The listing builds one solid part. Answer for the finished solid, in the listing's coordinates (mm). A direction names the side the tool comes from. Round coordinates to 2 decimals unless told otherwise and drop trailing zeros. Write each loop counter-clockwise with the first axis right and the second up, starting at its lowest first coordinate (ties: lowest second). Pieces come first, ordered by that corner, then holes.
(1) The mould has two halves that part along Y. Classify faces 5 (the face through (7.013, -0.356, 44.539)), 6 (the face through (72.38, 21.78, 6.44)), 7 (the face through (72.38, -21.78, 6.44)), 8 (the face through (29.1, -2.93, 7.066)): +Y half, -Y half, draft (parallel to the pull), parting line (faces both ways), or undercut.
(2) A cutting plane is placed at A-A, the plane x = 27. Give the vertices of the cut face in (y, z).
(3) A cutting plane is placed at D-D, the plane y = -9. Give the vertices of the cut face in (x, z).
(4) Find the intervals of material crossed by probe 1 along Z at (x, y) = (28, 0); probe 2 along Z at (x, y) = (43, 0); probe 3 along X at (y, z) = (8.5, 15), in increasing order.
(5) A cutting plane is placed at C-C, the plane z = 36. Give the vertices of the cut face in (x, y), and give its area (3 significant figures).
(6) A cutting plane is placed at B-B, the plane y = 0. Give the vertices of the cut face in (x, z), and give its area (3 significant figures).
(7) For faces 1 (the face through (25.4, -19, 38)), 2 (the face through (25.4, 19, 38)), 3 (the face through (24, -25.4, 20)), 4 (the face through (64, 16, 12.7)), determine the directions among +Z, -Z, +X, -X, +Y, -Y from which every point of the face is accessible in a straight line to the end or side of a thin tool.
(8) Each of these flat-tipped pins is pushed along its axis until it touches: pin 1 Ø20.5 at (x, z) = (34.5, 32.5) entering from +Y; pin 2 Ø12.5 at (x, z) = (40.5, 35.5) entering from -Y; pin 3 Ø4 at (x, y) = (32, -20) entering from +Z; pin 4 Ø6.5 at (x, y) = (45.5, -4) entering from +Z. Where does it stop, or does it pass through?
from build123d import *

# Parameters (mm, degrees)
F1_DEPTH = 25.4
F2_DEPTH = 12.7
F3_R     = 6.35
F4_DEPTH = 76.201
F5_R     = 12.7


with BuildPart() as f1:
    # F0 (on Front) → F1 (new body, symmetric)
    with BuildSketch(Plane.XZ):
        Polygon((0, 38.1), (0, 0), (76.2, 0), (76.2, 12.7), (50.8, 12.7), (50.8, 25.4), (25.4, 25.4), (25.4, 50.8), (13.832867, 50.8), align=None)
    extrude(amount=F1_DEPTH, both=True)

    # F0 (on Front) → F2 (join, symmetric)
    with BuildSketch(Plane.XZ):
        Polygon((38.1, 50.8), (25.4, 50.8), (25.4, 25.4), (50.8, 25.4), (50.8, 38.1), (38.1, 38.1), align=None)
    extrude(amount=F2_DEPTH, both=True)

    # F3 (on face) → F4 (cut, through all)
    with BuildSketch(Plane(origin=(0, 0, 0), x_dir=(0, -1, 0), z_dir=(-1, 0, 0))):
        with Locations((0, 12.7)):
            Circle(F3_R)
    extrude(amount=-F4_DEPTH, mode=Mode.SUBTRACT)

    # F5
    f5_edges = [f1.edges().sort_by_distance(p)[0] for p in [
        (76.2, 25.4, 6.35),
        (76.2, -25.4, 6.35),
    ]]
    fillet(f5_edges, radius=F5_R)


solid = f1.part
Solutions:
1. face 5: draft
1. face 6: +Y half
1. face 7: -Y half
1. face 8: undercut
2. outline: (-25.4, 0) - (25.4, 0) - (25.4, 25.4) - (12.7, 25.4) - (12.7, 50.8) - (-12.7, 50.8) - (-12.7, 25.4) - (-25.4, 25.4) - close; hole circle Ø12.7 at (0, 12.7)
3. outline: (0, 0) - (76.2, 0) - (76.2, 12.7) - (50.8, 12.7) - (50.8, 38.1) - (38.1, 38.1) - (38.1, 50.8) - (13.83, 50.8) - (0, 38.1) - close
4. probe 1: z = 0 to 6.35, 19.05 to 50.8
4. probe 2: z = 0 to 6.35, 19.05 to 38.1
4. probe 3: x = 0 to 50.8
5. outline: (0, -25.4) - (25.4, -25.4) - (25.4, -12.7) - (50.8, -12.7) - (50.8, 12.7) - (25.4, 12.7) - (25.4, 25.4) - (0, 25.4) - close
5. area: 1,940 mm2
6. outline: (0, 0) - (76.2, 0) - (76.2, 6.35) - (0, 6.35) - close; (0, 19.05) - (50.8, 19.05) - (50.8, 38.1) - (38.1, 38.1) - (38.1, 50.8) - (13.83, 50.8) - (0, 38.1) - close
6. area: 1,850 mm2
7. face 1: +Z, +X, -Y
7. face 2: +Z, +X, +Y
7. face 3: +Z, -Z, +X, -X, -Y
7. face 4: +Z, +X, +Y, -Y
8. pin 1: stops at y = 25.4
8. pin 2: stops at y = -12.7
8. pin 3: stops at z = 25.4
8. pin 4: stops at z = 38.1
